Part model, mm, in its own coordinate system. A direction names the side the tool comes from. Coordinates: 2 decimals unless noted, no trailing zeros. Write each loop counter-clockwise with the first axis right and the second up, starting at its lowest first coordinate (ties: lowest second). Pieces come first, ordered by that corner, then holes. Notation, with made-up numbers: M 46.25,-18 L 72.25,-18 A28 ccw 72.25,10 Z; hole C 72,64 d10. An arc over 180 degrees is marked long. Use a Markdown table: item, result. Add a question column.
Q1. Pin check, flat tips, straight feed: pin 1 Ø1.5 at (x, z) = (-1, 8) entering from +Y; pin 2 Ø0.8 at (x, z) = (-0.5, 28.5) entering from +Y. Stop position of each tip, or through.
Q2. Slice it at D-D on y = 1.05. Write the cut outline in (x, z).
Q3. Slice it at B-B on z = 3.25. Write the cut outline in (x, y) (1 decimal).
Q4. Mould opens along Y. For faces 1 (the flat face through (0, 0.4, 0)), 2 (the flat face through (0, 0, 3)), 3 (the flat face through (0, 0, 27)), 4 (the cylindrical face through (-0.34, -1.55, 12.52)) say: released by +Y, released by -Y, zero draft, split by the parting line, or undercut.
Q5. Slice it at C-C on z = 25. Write the cut outline in (x, y) (1 decimal), then the cut area to 3 significant figures.
Q6. Tool access for faces 5 (the flat face through (0, -1, 6)), 6 (the cylindrical face through (-0.027, -1.224, 27.372)), 7 (the flat face through (0, -0.5, 29.4)): list every direction of +Z, -Z, +X, -X, +Y, -Y with a clear straight run to the whole face (end or side of a thin tool).
Q7. Slice it at A-A on x = 0. Write the cut outline in (y, z), then the cut area to 3 significant figures.
Q8. Wall check: L1, parallel to Z at x = 0, y = -0.35; L2, parallel to Z at x = 1.1, y = 1; L3, parallel to X at y = 0.65, z = 13. Give the ranges that are in metal, low to high. Write a range as from..to.
from build123d import *

# Parameters (mm, degrees)
F0_R     = 1.5875
F1_DEPTH = 25.4
F3_DEPTH = 4
F5_DEPTH = 6


with BuildPart() as f1:
    # F0 (on Top) → F1 (new body)
    with BuildSketch(Plane.XY):
        Circle(F0_R)
    extrude(amount=F1_DEPTH)

    # F2 (on face) → F3 (join)
    with BuildSketch(Plane.XY.offset(25.4)):
        with BuildLine():
            ThreePointArc((-1.269985, 0), (0, -1.224553), (1.269985, 0))
            Line((1.269985, 0), (-1.269985, 0))
        make_face()
    extrude(amount=F3_DEPTH)

    # F4 (on face) → F5 (cut)
    with BuildSketch(Plane(origin=(0, 0, 0), x_dir=(1, 0, 0), z_dir=(0, 0, -1))):
        with BuildLine():
            ThreePointArc((1.27, 0), (0, 1.27), (-1.27, 0))
            Line((-1.27, 0), (1.27, 0))
        make_face()
    extrude(amount=-F5_DEPTH, mode=Mode.SUBTRACT)


solid = f1.part
Recorded:
| question | item | result |
|---|---|---|
| 1 | pin 1 | y = 1.57 |
| 1 | pin 2 | y = 0 |
| 2 | outline | M -1.19,0 L 1.19,0 L 1.19,25.4 L -1.19,25.4 Z |
| 3 | outline | C 0,0 d3.2; hole M -1.3,0 A1.3 ccw 1.3,0 Z |
| 4 | face 1 | zero draft |
| 4 | face 2 | undercut |
| 4 | face 3 | released by +Y |
| 4 | face 4 | split by the parting line |
| 5 | outline | C 0,0 d3.2 |
| 5 | area | 7.92 mm² |
| 6 | face 5 | -Z |
| 6 | face 6 | +Z, -Y |
| 6 | face 7 | +Z, +X, -X, +Y, -Y |
| 7 | outline | M -1.59,0 L -1.27,0 L -1.27,6 L 0,6 L 0,0 L 1.59,0 L 1.59,25.4 L 0,25.4 L 0,29.4 L -1.22,29.4 L -1.22,25.4 L -1.59,25.4 Z |
| 7 | area | 77.9 mm² |
| 8 | L1 | 6..29.4 |
| 8 | L2 | 0..25.4 |
| 8 | L3 | -1.45..1.45 |
